For this review, take the finished solid that the model builds, in its own axes (mm). Round coordinates to 2 decimals unless told otherwise and drop trailing zeros. Use a Markdown table: item, result. Add a question column.
1) Consider section A-A (z = 511). Give the number of separate pieces and of enclosed holes in the cut face, plus the area to 3 significant figures.
2) Wall thickness on line 1 along X through (y, z) = (-18.5, 165.5); line 2 along X through (y, z) = (0, 178); line 3 along Y through (x, z) = (-22.5, 383): over which ranges is each line inside the solid? List them lowest first. Write a range as [from, to].
3) Clearance check with flat-ended pins moving along their axes: P1, Ø3.5, axis at y = -23, z = 261, coming from the +X side; P2, Ø0.6, axis at y = -24.5, z = 393, coming from the -X side; P3, Ø3, axis at x = -11.5, z = 118.5, coming from the +Y side; P4, Ø1.5, axis at x = -18.5, y = -4.5, coming from the -Z side. State where each tip first meets the part, or that it passes through.
```python
from build123d import *

# Parameters (mm, degrees)
SKETCH_1_R      = 3.4
EXTRUDE_1_DEPTH = 795


with BuildPart() as part:
    # 草图1 → 凸台-拉伸1 (new body)
    with BuildSketch(Plane.XY):
        with BuildLine():
            Line((-1.911920332, 0.735190406), (2.405846621, 5.052957359))
            Line((2.405846621, 5.052957359), (7.388079668, 5.052957359))
            ThreePointArc((7.388079668, 5.052957359), (8.09518645, 4.76006414), (8.388079668, 4.052957359))
            Line((8.388079668, 4.052957359), (8.388079668, 2.402957359))
            ThreePointArc((8.388079668, 2.402957359), (8.09518645, 1.695850578), (7.388079668, 1.402957359))
            Line((7.388079668, 1.402957359), (5.888079668, 1.402957359))
            Line((5.888079668, 1.402957359), (5.888079668, -0.797042641))
            ThreePointArc((5.888079668, -0.797042641), (5.975947634, -1.009174675), (6.188079668, -1.097042641))
            Line((6.188079668, -1.097042641), (9.388079668, -1.097042641))
            Line((9.388079668, -1.097042641), (9.388079668, -0.297042641))
            ThreePointArc((9.388079668, -0.297042641), (9.446658312, -0.155621285), (9.588079668, -0.097042641))
            Line((9.588079668, -0.097042641), (10.388079668, -0.097042641))
            Line((10.388079668, -0.097042641), (10.388079668, 10.302957359))
            ThreePointArc((10.388079668, 10.302957359), (9.070060184, 13.484937874), (5.888079668, 14.802957359))
            Line((5.888079668, 14.802957359), (-4.511920332, 14.802957359))
            Line((-4.511920332, 14.802957359), (-4.511920332, 14.002957359))
            ThreePointArc((-4.511920332, 14.002957359), (-4.570498975, 13.861536003), (-4.711920332, 13.802957359))
            Line((-4.711920332, 13.802957359), (-5.511920332, 13.802957359))
            Line((-5.511920332, 13.802957359), (-5.511920332, 10.602957359))
            ThreePointArc((-5.511920332, 10.602957359), (-5.424052366, 10.390825325), (-5.211920332, 10.302957359))
            Line((-5.211920332, 10.302957359), (-3.011920332, 10.302957359))
            Line((-3.011920332, 10.302957359), (-3.011920332, 11.802957359))
            ThreePointArc((-3.011920332, 11.802957359), (-2.719027113, 12.51006414), (-2.011920332, 12.802957359))
            Line((-2.011920332, 12.802957359), (-0.361920332, 12.802957359))
            ThreePointArc((-0.361920332, 12.802957359), (0.34518645, 12.51006414), (0.638079668, 11.802957359))
            Line((0.638079668, 11.802957359), (0.638079668, 6.820724312))
            Line((0.638079668, 6.820724312), (-3.679687285, 2.502957359))
            Line((-3.679687285, 2.502957359), (-15.544153379, 2.502957359))
            Line((-15.544153379, 2.502957359), (-19.861920332, 6.820724312))
            Line((-19.861920332, 6.820724312), (-19.861920332, 11.802957359))
            ThreePointArc((-19.861920332, 11.802957359), (-19.569027113, 12.51006414), (-18.861920332, 12.802957359))
            Line((-18.861920332, 12.802957359), (-17.211920332, 12.802957359))
            ThreePointArc((-17.211920332, 12.802957359), (-16.50481355, 12.51006414), (-16.211920332, 11.802957359))
            Line((-16.211920332, 11.802957359), (-16.211920332, 10.302957359))
            Line((-16.211920332, 10.302957359), (-14.011920332, 10.302957359))
            ThreePointArc((-14.011920332, 10.302957359), (-13.799788297, 10.390825325), (-13.711920332, 10.602957359))
            Line((-13.711920332, 10.602957359), (-13.711920332, 13.802957359))
            Line((-13.711920332, 13.802957359), (-14.511920332, 13.802957359))
            ThreePointArc((-14.511920332, 13.802957359), (-14.653341688, 13.861536003), (-14.711920332, 14.002957359))
            Line((-14.711920332, 14.002957359), (-14.711920332, 14.802957359))
            Line((-14.711920332, 14.802957359), (-25.111920332, 14.802957359))
            ThreePointArc((-25.111920332, 14.802957359), (-28.293900847, 13.484937874), (-29.611920332, 10.302957359))
            Line((-29.611920332, 10.302957359), (-29.611920332, -0.097042641))
            Line((-29.611920332, -0.097042641), (-28.811920332, -0.097042641))
            ThreePointArc((-28.811920332, -0.097042641), (-28.670498975, -0.155621285), (-28.611920332, -0.297042641))
            Line((-28.611920332, -0.297042641), (-28.611920332, -1.097042641))
            Line((-28.611920332, -1.097042641), (-25.411920332, -1.097042641))
            ThreePointArc((-25.411920332, -1.097042641), (-25.199788297, -1.009174675), (-25.111920332, -0.797042641))
            Line((-25.111920332, -0.797042641), (-25.111920332, 1.402957359))
            Line((-25.111920332, 1.402957359), (-26.611920332, 1.402957359))
            ThreePointArc((-26.611920332, 1.402957359), (-27.319027113, 1.695850578), (-27.611920332, 2.402957359))
            Line((-27.611920332, 2.402957359), (-27.611920332, 4.052957359))
            ThreePointArc((-27.611920332, 4.052957359), (-27.319027113, 4.76006414), (-26.611920332, 5.052957359))
            Line((-26.611920332, 5.052957359), (-21.629687285, 5.052957359))
            Line((-21.629687285, 5.052957359), (-17.311920332, 0.735190406))
            Line((-17.311920332, 0.735190406), (-17.311920332, -11.129275688))
            Line((-17.311920332, -11.129275688), (-21.629687285, -15.447042641))
            Line((-21.629687285, -15.447042641), (-26.611920332, -15.447042641))
            ThreePointArc((-26.611920332, -15.447042641), (-27.319027113, -15.154149422), (-27.611920332, -14.447042641))
            Line((-27.611920332, -14.447042641), (-27.611920332, -12.797042641))
            ThreePointArc((-27.611920332, -12.797042641), (-27.319027113, -12.08993586), (-26.611920332, -11.797042641))
            Line((-26.611920332, -11.797042641), (-25.111920332, -11.797042641))
            Line((-25.111920332, -11.797042641), (-25.111920332, -9.597042641))
            ThreePointArc((-25.111920332, -9.597042641), (-25.199788297, -9.384910607), (-25.411920332, -9.297042641))
            Line((-25.411920332, -9.297042641), (-28.611920332, -9.297042641))
            Line((-28.611920332, -9.297042641), (-28.611920332, -10.097042641))
            ThreePointArc((-28.611920332, -10.097042641), (-28.670498975, -10.238463997), (-28.811920332, -10.297042641))
            Line((-28.811920332, -10.297042641), (-29.611920332, -10.297042641))
            Line((-29.611920332, -10.297042641), (-29.611920332, -20.697042641))
            ThreePointArc((-29.611920332, -20.697042641), (-28.293900847, -23.879023156), (-25.111920332, -25.197042641))
            Line((-25.111920332, -25.197042641), (-14.711920332, -25.197042641))
            Line((-14.711920332, -25.197042641), (-14.711920332, -24.397042641))
            ThreePointArc((-14.711920332, -24.397042641), (-14.653341688, -24.255621285), (-14.511920332, -24.197042641))
            Line((-14.511920332, -24.197042641), (-13.711920332, -24.197042641))
            Line((-13.711920332, -24.197042641), (-13.711920332, -20.997042641))
            ThreePointArc((-13.711920332, -20.997042641), (-13.799788297, -20.784910607), (-14.011920332, -20.697042641))
            Line((-14.011920332, -20.697042641), (-16.211920332, -20.697042641))
            Line((-16.211920332, -20.697042641), (-16.211920332, -22.197042641))
            ThreePointArc((-16.211920332, -22.197042641), (-16.50481355, -22.904149422), (-17.211920332, -23.197042641))
            Line((-17.211920332, -23.197042641), (-18.861920332, -23.197042641))
            ThreePointArc((-18.861920332, -23.197042641), (-19.569027113, -22.904149422), (-19.861920332, -22.197042641))
            Line((-19.861920332, -22.197042641), (-19.861920332, -17.214809594))
            Line((-19.861920332, -17.214809594), (-15.544153379, -12.897042641))
            Line((-15.544153379, -12.897042641), (-3.679687285, -12.897042641))
            Line((-3.679687285, -12.897042641), (0.638079668, -17.214809594))
            Line((0.638079668, -17.214809594), (0.638079668, -22.197042641))
            ThreePointArc((0.638079668, -22.197042641), (0.34518645, -22.904149422), (-0.361920332, -23.197042641))
            Line((-0.361920332, -23.197042641), (-2.011920332, -23.197042641))
            ThreePointArc((-2.011920332, -23.197042641), (-2.719027113, -22.904149422), (-3.011920332, -22.197042641))
            Line((-3.011920332, -22.197042641), (-3.011920332, -20.697042641))
            Line((-3.011920332, -20.697042641), (-5.211920332, -20.697042641))
            ThreePointArc((-5.211920332, -20.697042641), (-5.424052366, -20.784910607), (-5.511920332, -20.997042641))
            Line((-5.511920332, -20.997042641), (-5.511920332, -24.197042641))
            Line((-5.511920332, -24.197042641), (-4.711920332, -24.197042641))
            ThreePointArc((-4.711920332, -24.197042641), (-4.570498975, -24.255621285), (-4.511920332, -24.397042641))
            Line((-4.511920332, -24.397042641), (-4.511920332, -25.197042641))
            Line((-4.511920332, -25.197042641), (5.888079668, -25.197042641))
            ThreePointArc((5.888079668, -25.197042641), (9.070060184, -23.879023156), (10.388079668, -20.697042641))
            Line((10.388079668, -20.697042641), (10.388079668, -10.297042641))
            Line((10.388079668, -10.297042641), (9.588079668, -10.297042641))
            ThreePointArc((9.588079668, -10.297042641), (9.446658312, -10.238463997), (9.388079668, -10.097042641))
            Line((9.388079668, -10.097042641), (9.388079668, -9.297042641))
            Line((9.388079668, -9.297042641), (6.188079668, -9.297042641))
            ThreePointArc((6.188079668, -9.297042641), (5.975947634, -9.384910607), (5.888079668, -9.597042641))
            Line((5.888079668, -9.597042641), (5.888079668, -11.797042641))
            Line((5.888079668, -11.797042641), (7.388079668, -11.797042641))
            ThreePointArc((7.388079668, -11.797042641), (8.09518645, -12.08993586), (8.388079668, -12.797042641))
            Line((8.388079668, -12.797042641), (8.388079668, -14.447042641))
            ThreePointArc((8.388079668, -14.447042641), (8.09518645, -15.154149422), (7.388079668, -15.447042641))
            Line((7.388079668, -15.447042641), (2.405846621, -15.447042641))
            Line((2.405846621, -15.447042641), (-1.911920332, -11.129275688))
            Line((-1.911920332, -11.129275688), (-1.911920332, 0.735190406))
        make_face()
        with Locations((-9.611920332, -5.197042641)):
            Circle(SKETCH_1_R, mode=Mode.SUBTRACT)
        with BuildLine():
            Line((3.138079668, -16.947042641), (7.892079668, -16.947042641))
            ThreePointArc((7.892079668, -16.947042641), (8.59918645, -17.23993586), (8.892079668, -17.947042641))
            Line((8.892079668, -17.947042641), (8.892079668, -21.201042641))
            ThreePointArc((8.892079668, -21.201042641), (8.159846621, -22.968809594), (6.392079668, -23.701042641))
            Line((6.392079668, -23.701042641), (3.138079668, -23.701042641))
            ThreePointArc((3.138079668, -23.701042641), (2.430972887, -23.408149422), (2.138079668, -22.701042641))
            Line((2.138079668, -22.701042641), (2.138079668, -17.947042641))
            ThreePointArc((2.138079668, -17.947042641), (2.430972887, -17.23993586), (3.138079668, -16.947042641))
        make_face(mode=Mode.SUBTRACT)
        with BuildLine():
            Line((-21.361920332, -17.947042641), (-21.361920332, -22.701042641))
            ThreePointArc((-21.361920332, -22.701042641), (-21.65481355, -23.408149422), (-22.361920332, -23.701042641))
            Line((-22.361920332, -23.701042641), (-25.615920332, -23.701042641))
            ThreePointArc((-25.615920332, -23.701042641), (-27.383687285, -22.968809594), (-28.115920332, -21.201042641))
            Line((-28.115920332, -21.201042641), (-28.115920332, -17.947042641))
            ThreePointArc((-28.115920332, -17.947042641), (-27.823027113, -17.23993586), (-27.115920332, -16.947042641))
            Line((-27.115920332, -16.947042641), (-22.361920332, -16.947042641))
            ThreePointArc((-22.361920332, -16.947042641), (-21.65481355, -17.23993586), (-21.361920332, -17.947042641))
        make_face(mode=Mode.SUBTRACT)
        with BuildLine():
            Line((2.138079668, 7.552957359), (2.138079668, 12.306957359))
            ThreePointArc((2.138079668, 12.306957359), (2.430972887, 13.01406414), (3.138079668, 13.306957359))
            Line((3.138079668, 13.306957359), (6.392079668, 13.306957359))
            ThreePointArc((6.392079668, 13.306957359), (8.159846621, 12.574724312), (8.892079668, 10.806957359))
            Line((8.892079668, 10.806957359), (8.892079668, 7.552957359))
            ThreePointArc((8.892079668, 7.552957359), (8.59918645, 6.845850578), (7.892079668, 6.552957359))
            Line((7.892079668, 6.552957359), (3.138079668, 6.552957359))
            ThreePointArc((3.138079668, 6.552957359), (2.430972887, 6.845850578), (2.138079668, 7.552957359))
        make_face(mode=Mode.SUBTRACT)
        with BuildLine():
            Line((-22.361920332, 6.552957359), (-27.115920332, 6.552957359))
            ThreePointArc((-27.115920332, 6.552957359), (-27.823027113, 6.845850578), (-28.115920332, 7.552957359))
            Line((-28.115920332, 7.552957359), (-28.115920332, 10.806957359))
            ThreePointArc((-28.115920332, 10.806957359), (-27.383687285, 12.574724312), (-25.615920332, 13.306957359))
            Line((-25.615920332, 13.306957359), (-22.361920332, 13.306957359))
            ThreePointArc((-22.361920332, 13.306957359), (-21.65481355, 13.01406414), (-21.361920332, 12.306957359))
            Line((-21.361920332, 12.306957359), (-21.361920332, 7.552957359))
            ThreePointArc((-21.361920332, 7.552957359), (-21.65481355, 6.845850578), (-22.361920332, 6.552957359))
        make_face(mode=Mode.SUBTRACT)
    extrude(amount=EXTRUDE_1_DEPTH)


solid = part.part
```
Results list:
| question | item | result |
|---|---|---|
| 1 | separate pieces | 1 |
| 1 | enclosed holes | 5 |
| 1 | area | 581 mm2 |
| 2 | line 1 | [-29.61, -28.12], [-21.36, -19.86], [0.64, 2.14], [8.89, 10.39] |
| 2 | line 2 | [-29.61, -25.11], [-17.31, -1.91], [5.89, 10.39] |
| 2 | line 3 | [-25.2, -23.7], [-16.95, -15.45], [5.05, 6.55], [13.31, 14.8] |
| 3 | P1 | x = 10.35 |
| 3 | P2 | x = -27.94 |
| 3 | P3 | y = 2.5 |
| 3 | P4 | through |
